from build123d import *

# Parameters (mm, degrees)
SKETCH_1_R      = 41
SKETCH_1_R_2    = 1.525
EXTRUDE_1_DEPTH = 2
EXTRUDE_3_DEPTH = 2
FILLET_1_R      = 2
FILLET_2_R      = 2
EXTRUDE_5_DEPTH = 1.5
FILLET_3_R      = 2


with BuildPart() as part:
    # 草图1 → 凸台-拉伸1 (new body)
    with BuildSketch(Plane(origin=(0, 0, 0), x_dir=(1, 0, 0), z_dir=(0, 1, 0))):
        with BuildLine():
            Line((-54, 0), (-54, 54))
            Line((-54, 54), (-10, 54))
            Line((-10, 54), (-10, 53.065996646))
            ThreePointArc((-10, 53.065996646), (41.569219382, -34.467375879), (-54, 0))
        make_face()
        with Locations(Location((0, 0, 0), (0, 0, 270))):
            Circle(SKETCH_1_R, mode=Mode.SUBTRACT)
        with Locations(Location((-15, 46.647615159, 0), (0, 0, 270))):
            Circle(SKETCH_1_R_2, mode=Mode.SUBTRACT)
        with Locations(Location((0, 49, 0), (0, 0, 270))):
            Circle(SKETCH_1_R_2, mode=Mode.SUBTRACT)
        with Locations(Location((49, 0, 0), (0, 0, 270))):
            Circle(SKETCH_1_R_2, mode=Mode.SUBTRACT)
        with Locations(Location((0, -49, 0), (0, 0, 270))):
            Circle(SKETCH_1_R_2, mode=Mode.SUBTRACT)
        with Locations(Location((-49, 0, 0), (0, 0, 270))):
            Circle(SKETCH_1_R_2, mode=Mode.SUBTRACT)
        with Locations(Location((-49, 46.647615159, 0), (0, 0, 270))):
            Circle(SKETCH_1_R_2, mode=Mode.SUBTRACT)
    extrude(amount=EXTRUDE_1_DEPTH)

    # 草图2 → 凸台-拉伸3 (add)
    with BuildSketch(Plane(origin=(0, 0, 0), x_dir=(1, 0, 0), z_dir=(0, 1, 0))):
        with BuildLine():
            Line((-41, 0), (-37.46998799, 0))
            ThreePointArc((-37.46998799, 0), (-36.430757506, 0.418334617), (-35.971188471, 1.44))
            ThreePointArc((-35.971188471, 1.44), (-31.023847214, 18.262554696), (-18.716133348, 30.752338976))
            ThreePointArc((-18.716133348, 30.752338976), (-18.190087037, 31.295672989), (-17.99598895, 32.026605615))
            Line((-17.99598895, 32.026605615), (-17.973217018, 36.850555898))
            ThreePointArc((-17.973217018, 36.850555898), (-34.769971942, 21.726689834), (-41, 0))
        make_face()
    extrude(amount=EXTRUDE_3_DEPTH)

    # 圆角1
    fillet_1_edges = [part.edges().sort_by_distance(p)[0] for p in [
        (-17.973217018, 1, -36.850555898),
        (-41, 1, 0),
    ]]
    fillet(fillet_1_edges, radius=FILLET_1_R)

    # 圆角2
    # the kernel refuses this fillet: 2 mm, written as the material it adds along each edge
    with BuildSketch(Plane(origin=(-10, 0, -53.065996646), x_dir=(0, 0, -1), z_dir=(0, 1, 0))) as fillet_2_piece_1:
        with BuildLine():
            CenterArc((2.281728124, -1.477713756), FILLET_2_R, 132.365870045, 56.387625402)
            ThreePointArc((0.305023668, -1.782081122), (0.159970683, -0.889763893), (0, 0))
            Line((0, 0), (0.934003354, 0))
        make_face()
    extrude(amount=2)
    # the kernel refuses this fillet: 2 mm, written as the material it takes off along each edge
    with BuildSketch(Plane(origin=(-54, -5, -54), x_dir=(0, 0, 1), z_dir=(0, 1, 0))) as fillet_2_2_piece_1:
        with BuildLine():
            CenterArc((FILLET_2_R, FILLET_2_R), FILLET_2_R, 180, 90)
            Line((0, FILLET_2_R), (0, 0))
            Line((0, 0), (FILLET_2_R, 0))
        make_face()
    extrude(amount=12, mode=Mode.SUBTRACT)

    # 草图4 → 凸台-拉伸5 (add)
    with BuildSketch(Plane.XZ):
        with BuildLine():
            Line((-38.948684188, 0), (-37.46998799, 0))
            ThreePointArc((-37.46998799, 0), (-36.430757506, -0.418334617), (-35.971188471, -1.44))
            ThreePointArc((-35.971188471, -1.44), (-35.662320704, 4.919235918), (-34.238034587, 11.124611797))
            Line((-34.238034587, 11.124611797), (-38.993317168, 12.669696769))
            ThreePointArc((-38.993317168, 12.669696769), (-40.317388101, 7.450383664), (-40.946052608, 2.102564103))
            ThreePointArc((-40.946052608, 2.102564103), (-40.398706292, 0.622525537), (-38.948684188, 0))
        make_face()
    extrude(amount=-EXTRUDE_5_DEPTH)

    # 圆角3
    fillet_3_edges = [part.edges().sort_by_distance(p)[0] for p in [
        (-38.993317168, 0.75, 12.669696769),
        (-34.238034587, 0.75, 11.124611797),
    ]]
    fillet(fillet_3_edges, radius=FILLET_3_R)


solid = part.part
Part model, mm, in its own coordinate system. A direction names the side the tool comes from. Give positions to 0.01 mm unless a question says otherwise; leave off trailing zeros. Write each loop counter-clockwise with the first axis right and the second up, starting at its lowest first coordinate (ties: lowest second). Pieces come first, ordered by that corner, then holes.
1) Cut at B-B on z = 49. Write the cut outline in (x, y) (3 decimals), then the cut area to 3 significant figures.
Resolved:
outline: (-22.694, 0) - (-1.525, 0) - (-1.525, 2) - (-22.694, 2) - close; (1.525, 0) - (22.694, 0) - (22.694, 2) - (1.525, 2) - close
area: 84.7 mm2
2) Two-plate mould, pull along X, no slides. Class faces 1 (the face through (-37, 0, -11)), 2 (the face through (0.067, 0.986, -50.524)): released by +X, released by -X, zero draft, split by the parting line, or undercut.
Resolved:
face 1: zero draft
face 2: undercut
3) Pin check, flat tip, straight feed: pin 1 (3 mm diameter, centred on x = -38.5, z = 5.5, fed in from +Y). Stop position of the tip, or through.
Resolved:
pin 1: stops at y = 1.5
4) Cut at A-A on x = 7. Write the cut outline in (y, z).
Resolved:
outline: (0, -53.54) - (2, -53.54) - (2, -40.4) - (0, -40.4) - close; (0, 40.4) - (2, 40.4) - (2, 53.54) - (0, 53.54) - close
5) Which spindle directions (+Z, -Z, +X, -X, +Y, -Y) get a long thin tool onto all of the face, cutting with end or side? Do faces 3 (the face through (-15.928, 0.986, -47.858)), 4 (the face through (-38, 1.5, 7)). Say none if no direction does.
Resolved:
face 3: +Y, -Y
face 4: +Y
6) Cut at C-C on x = -49. Write the cut outline in (y, z) (3 decimals).
Resolved:
outline: (0, -54) - (2, -54) - (2, -48.173) - (0, -48.173) - close; (0, -45.123) - (2, -45.123) - (2, -1.525) - (0, -1.525) - close; (0, 1.525) - (2, 1.525) - (2, 22.694) - (0, 22.694) - close
7) Probe L1, parallel to X at y = 0.55, z = 0 (3 decimals); L2, parallel to Z at x = -14.5, y = 1.35; L3, parallel to X at y = 0.95, z = 1. List the from-to ranges inside material, lowest first.
Resolved:
L1: x = -54 to -50.525, -47.475 to -36, 41 to 47.475, 50.525 to 54
L2: z = -54 to -48.09, -45.21 to -38.35, 38.35 to 52.02
L3: x = -53.99 to -50.15, -47.85 to -35.99, 40.99 to 47.85, 50.15 to 53.99
8) Cut at D-D on y = 0.35. Write the cut outline in (x, z) (3 decimals).
Resolved:
outline: (-54, -52) arc R2 ccw to (-52, -54) - (-10, -54) arc R2 cw to (-8.218, -53.371) arc R54 ccw (long way) to (-54, 0) - close; hole circle Ø3.05 at (-49, -46.648); hole circle Ø3.05 at (-49, 0); hole (-38.292, 14.653) arc R2 ccw to (-37.042, 12.036) - (-36.09, 11.726) arc R2 cw to (-34.776, 9.307) arc R36 ccw to (-18.716, -30.752) arc R1.5 cw to (-17.996, -32.027) - (-17.979, -35.586) arc R2 ccw to (-16.799, -37.401) arc R41 ccw (long way) to start; hole circle Ø3.05 at (-15, -46.648); hole circle Ø3.05 at (0, -49); hole circle Ø3.05 at (0, 49); hole circle Ø3.05 at (49, 0)
